from build123d import *

# Parameters (mm, degrees)
BOSS_EXTRUDE1_DEPTH = 20
SKETCH2_R           = 2.2
CUT_EXTRUDE1_DEPTH  = 123.202659546
SKETCH3_R           = 8
BOSS_EXTRUDE2_DEPTH = 3
CUT_EXTRUDE2_REACH  = 129.16
SKETCH4_R           = 1.9
FILLET1_R           = 2
FILLET2_R           = 6


with BuildPart() as part:
    # Sketch1 → Boss-Extrude1 (new body)
    with BuildSketch(Plane.XY):
        Polygon((-25.4, 0), (25.4, 0), (25.4, 110.5), (28.4, 110.5), (28.4, -3), (19.3, -3), (19.3, -23), (16.3, -23), (16.3, -3), (-4.3, -3), (-4.3, -23), (-7.3, -23), (-7.3, -3), (-28.9, -3), (-28.9, 50), (-25.4, 50), align=None)
    extrude(amount=BOSS_EXTRUDE1_DEPTH)

    # Sketch2 → Cut-Extrude1 (cut, through all)
    with BuildSketch(Plane(origin=(19.3, 0, 0), x_dir=(0, 0, -1), z_dir=(1, 0, 0))):
        with Locations((-10, -13)):
            Circle(SKETCH2_R)
    extrude(amount=-CUT_EXTRUDE1_DEPTH, mode=Mode.SUBTRACT)

    # Sketch3 → Boss-Extrude2 (add)
    with BuildSketch(Plane(origin=(28.4, 0, 0), x_dir=(0, 0, -1), z_dir=(1, 0, 0))):
        with Locations((-18, 99.5)):
            Circle(SKETCH3_R)
        with Locations((-18, 15.5)):
            Circle(SKETCH3_R)
    extrude(amount=-BOSS_EXTRUDE2_DEPTH)

    # Sketch4 → Cut-Extrude2 (cut, up to next)
    with BuildSketch(Plane(origin=(28.4, 0, 0), x_dir=(0, 0, -1), z_dir=(1, 0, 0)), mode=Mode.PRIVATE) as cut_extrude2_sk1:
        with Locations(Location((-18, 99.5, 0), (0, 0, 90))):
            Circle(SKETCH4_R)
    cut_extrude2_tool1 = extrude(cut_extrude2_sk1.sketch, amount=-CUT_EXTRUDE2_REACH, mode=Mode.PRIVATE) & part.part
    # Sketch4 → Cut-Extrude2 (cut, up to next)
    with BuildSketch(Plane(origin=(28.4, 0, 0), x_dir=(0, 0, -1), z_dir=(1, 0, 0)), mode=Mode.PRIVATE) as cut_extrude2_sk2:
        with Locations(Location((-18, 15.5, 0), (0, 0, 90))):
            Circle(SKETCH4_R)
    cut_extrude2_tool2 = extrude(cut_extrude2_sk2.sketch, amount=-CUT_EXTRUDE2_REACH, mode=Mode.PRIVATE) & part.part
    add(cut_extrude2_tool1.solids().sort_by_distance((28.4, 99.5, 18))[0], mode=Mode.SUBTRACT)
    add(cut_extrude2_tool2.solids().sort_by_distance((28.4, 15.5, 18))[0], mode=Mode.SUBTRACT)

    # Fillet1
    fillet1_edges = [part.edges().sort_by_distance(p)[0] for p in [
        (26.9, 110.5, 0),
        (17.8, -23, 0),
        (-5.8, -23, 0),
        (-5.8, -23, 20),
        (-27.15, 50, 0),
        (25.4, 0, 10),
        (28.4, -3, 10),
        (19.3, -3, 10),
        (-7.3, -3, 10),
        (-28.9, -3, 10),
        (17.8, -23, 20),
        (26.9, 110.5, 20),
        (-27.15, 50, 20),
    ]]
    fillet(fillet1_edges, radius=FILLET1_R)

    # Fillet2
    fillet2_edges = [part.edges().sort_by_distance(p)[0] for p in [
        (26.9, 91.754033308, 20),
        (26.9, 107.245966692, 20),
        (26.9, 7.754033308, 20),
        (26.9, 23.245966692, 20),
    ]]
    fillet(fillet2_edges, radius=FILLET2_R)


solid = part.part
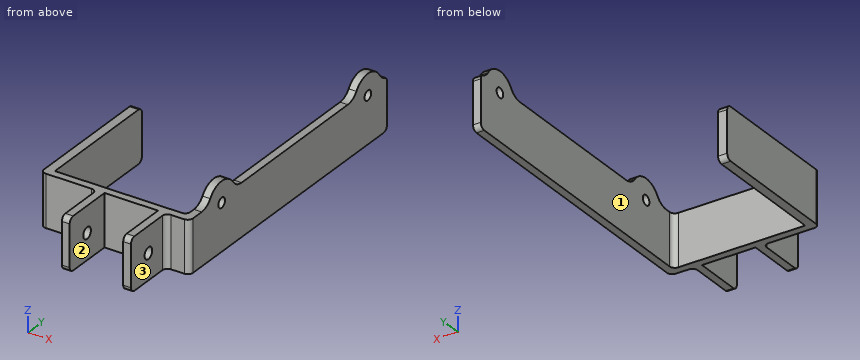
Model file for the job. Use its own axes, mm. Face numbers are marked on the shaded views. A direction names the side the tool comes from. Give positions to 0.01 mm unless a question says otherwise; leave off trailing zeros. Order: outer loops, then holes, each group sorted by start corner. A loop starts at its lowest first (then second) coordinate and runs counter-clockwise, first axis right, second up. Notation, with made-up numbers: M 88,-39 L 101,-39 A11 cw 101,-19 Z; hole C -14,72.25 d5. An arc over 180 degrees is marked long. Put each result on its own line as item: value. Start each with the question number.
(1) Band-saw the part on B-B on y = 15.5. Give the cut face in (x, z).
(2) Band-saw the part on D-D on y = 99. Give the cut face in (x, z).
(3) Drill centre lines: L1, parallel to Z at x = 27.5, y = 15.5; L2, parallel to Y at x = -6.6, z = 10; L3, parallel to X at y = 17, z = 15.25. Where is each one in solid material? Low to high. Write a range as [from, to].
(4) Band-saw the part on A-A on y = -13. Give the cut face in (x, z).
(5) Tool access for the marked faces 1, 2 and 3: list every direction of +Z, -Z, +X, -X, +Y, -Y with a clear straight run to the whole face (end or side of a thin tool).
(6) Pin check, flat tips, straight feed: pin 1 Ø1.5 at (x, y) = (27.5, 48.5) entering from +Z; pin 2 Ø5.5 at (y, z) = (-13, 10) entering from +X; pin 3 Ø4 at (y, z) = (90, 16.5) entering from -X. Stop position of each tip, or through.
(7) Band-saw the part on C-C on z = 4.5. Give the cut face in (x, y).
Results below:
1. outline: M -28.9,0 L -25.4,0 L -25.4,20 L -28.9,20 Z; M 25.4,0 L 28.4,0 L 28.4,16.1 L 25.4,16.1 Z; M 25.4,19.9 L 28.4,19.9 L 28.4,26 L 25.4,26 Z
2. outline: M 25.4,0 L 28.4,0 L 28.4,16.17 L 25.4,16.17 Z; M 25.4,19.83 L 28.4,19.83 L 28.4,25.98 L 25.4,25.98 Z
3. L1: z = [0, 16.1], [19.9, 26]
3. L2: y = [-23, -15.2], [-10.8, 0]
3. L3: x = [-28.9, -25.4], [25.4, 28.4]
4. outline: M -7.3,0 L -4.3,0 L -4.3,7.8 L -7.3,7.8 Z; M -7.3,12.2 L -4.3,12.2 L -4.3,20 L -7.3,20 Z; M 16.3,0 L 19.3,0 L 19.3,7.8 L 16.3,7.8 Z; M 16.3,12.2 L 19.3,12.2 L 19.3,20 L 16.3,20 Z
5. face 1: +Z, -Z, +Y
5. face 2: +Z, -Z, -Y
5. face 3: +Z, -Z, +X, -Y
6. pin 1: stops at z = 20
6. pin 2: stops at x = 19.3
6. pin 3: stops at x = 25.4
7. outline: M -28.9,-1 A2 ccw -26.9,-3 L -9.3,-3 A2 cw -7.3,-5 L -7.3,-23 L -4.3,-23 L -4.3,-3 L 16.3,-3 L 16.3,-23 L 19.3,-23 L 19.3,-5 A2 cw 21.3,-3 L 26.4,-3 A2 ccw 28.4,-1 L 28.4,110.5 L 25.4,110.5 L 25.4,2 A2 cw 23.4,0 L -25.4,0 L -25.4,50 L -28.9,50 Z
